from build123d import *

# Parameters (mm, degrees)
ESBO_O2_W                = 65.45
ESBO_O2_H                = 74.6
ESBO_O2_R                = 1.75
RESSALTO_EXTRUS_O1_DEPTH = 14.5
CORTE_EXTRUS_O1_REACH    = 84.743
ESBO_O3_W                = 6.5
ESBO_O3_H                = 12.9
ESBO_O4_W                = 48
ESBO_O4_H                = 74.6
RESSALTO_EXTRUS_O2_DEPTH = 4.5
ESBO_O5_W                = 20.2
ESBO_O5_H                = 12.15
ESBO_O5_W_2              = 30.35
RESSALTO_EXTRUS_O3_DEPTH = 8
ESBO_O6_R                = 4
RESSALTO_EXTRUS_O4_DEPTH = 12
FILETE1_R                = 0.8
CORTE_EXTRUS_O2_REACH    = 86.916
ESBO_O7_W                = 40.368182155
ESBO_O7_H                = 2.522042385
ESBO_O8_W                = 58.468294986
ESBO_O8_H                = 2.522042385
CORTE_EXTRUS_O3_DEPTH    = 71.953968353
ESBO_O9_W                = 3.722226521
ESBO_O9_H                = 2.522042385
ESBO_O9_W_2              = 3.909591324
CORTE_EXTRUS_O4_DEPTH    = 4
ESBO_O10_W               = 3.909591324
ESBO_O10_H               = 2.522042385
ESBO_O10_W_2             = 3.722226521
CORTE_EXTRUS_O5_DEPTH    = 3
FILETE2_R                = 1.5
FILETE3_R                = 0.3
ESBO_O11_W               = 9.960941138
ESBO_O11_H               = 18.14579458
RESSALTO_EXTRUS_O5_DEPTH = 6
ESBO_O12_W               = 18.14579458
ESBO_O12_H               = 6.154854005
CORTE_EXTRUS_O6_DEPTH    = 0.1
FILETE4_R                = 0.3


with BuildPart() as part:
    # Esboço2 → Ressalto-extrusão1 (new body)
    with BuildSketch(Plane(origin=(0, 0, 0), x_dir=(1, 0, 0), z_dir=(0, 1, 0))):
        Rectangle(ESBO_O2_W, ESBO_O2_H)
        with Locations(Location((27.725, 32.8, 0), (0, 0, 270))):
            Circle(ESBO_O2_R, mode=Mode.SUBTRACT)
        with Locations(Location((-27.725, 32.8, 0), (0, 0, 270))):
            Circle(ESBO_O2_R, mode=Mode.SUBTRACT)
        with Locations(Location((27.725, -32.8, 0), (0, 0, 270))):
            Circle(ESBO_O2_R, mode=Mode.SUBTRACT)
        with Locations(Location((-27.725, -32.8, 0), (0, 0, 270))):
            Circle(ESBO_O2_R, mode=Mode.SUBTRACT)
    extrude(amount=-RESSALTO_EXTRUS_O1_DEPTH)

    # Esboço3 → Corte-extrusão1 (cut, up to next)
    with BuildSketch(Plane(origin=(0, 0, -37.3), x_dir=(-1, 0, 0), z_dir=(0, 0, -1)), mode=Mode.PRIVATE) as corte_extrus_o1_sk1:
        with Locations((-27.975, -8.05)):
            Rectangle(ESBO_O3_W, ESBO_O3_H)
    corte_extrus_o1_tool1 = extrude(corte_extrus_o1_sk1.sketch, amount=-CORTE_EXTRUS_O1_REACH, mode=Mode.PRIVATE) & part.part
    # Esboço3 → Corte-extrusão1 (cut, up to next)
    with BuildSketch(Plane(origin=(0, 0, -37.3), x_dir=(-1, 0, 0), z_dir=(0, 0, -1)), mode=Mode.PRIVATE) as corte_extrus_o1_sk2:
        with Locations((-19.975, -8.05)):
            Rectangle(ESBO_O3_W, ESBO_O3_H)
    corte_extrus_o1_tool2 = extrude(corte_extrus_o1_sk2.sketch, amount=-CORTE_EXTRUS_O1_REACH, mode=Mode.PRIVATE) & part.part
    # Esboço3 → Corte-extrusão1 (cut, up to next)
    with BuildSketch(Plane(origin=(0, 0, -37.3), x_dir=(-1, 0, 0), z_dir=(0, 0, -1)), mode=Mode.PRIVATE) as corte_extrus_o1_sk3:
        with Locations((-11.975, -8.05)):
            Rectangle(ESBO_O3_W, ESBO_O3_H)
    corte_extrus_o1_tool3 = extrude(corte_extrus_o1_sk3.sketch, amount=-CORTE_EXTRUS_O1_REACH, mode=Mode.PRIVATE) & part.part
    # Esboço3 → Corte-extrusão1 (cut, up to next)
    with BuildSketch(Plane(origin=(0, 0, -37.3), x_dir=(-1, 0, 0), z_dir=(0, 0, -1)), mode=Mode.PRIVATE) as corte_extrus_o1_sk4:
        with Locations((-3.975, -8.05)):
            Rectangle(ESBO_O3_W, ESBO_O3_H)
    corte_extrus_o1_tool4 = extrude(corte_extrus_o1_sk4.sketch, amount=-CORTE_EXTRUS_O1_REACH, mode=Mode.PRIVATE) & part.part
    # Esboço3 → Corte-extrusão1 (cut, up to next)
    with BuildSketch(Plane(origin=(0, 0, -37.3), x_dir=(-1, 0, 0), z_dir=(0, 0, -1)), mode=Mode.PRIVATE) as corte_extrus_o1_sk5:
        with Locations((4.025, -8.05)):
            Rectangle(ESBO_O3_W, ESBO_O3_H)
    corte_extrus_o1_tool5 = extrude(corte_extrus_o1_sk5.sketch, amount=-CORTE_EXTRUS_O1_REACH, mode=Mode.PRIVATE) & part.part
    # Esboço3 → Corte-extrusão1 (cut, up to next)
    with BuildSketch(Plane(origin=(0, 0, -37.3), x_dir=(-1, 0, 0), z_dir=(0, 0, -1)), mode=Mode.PRIVATE) as corte_extrus_o1_sk6:
        with Locations((12.025, -8.05)):
            Rectangle(ESBO_O3_W, ESBO_O3_H)
    corte_extrus_o1_tool6 = extrude(corte_extrus_o1_sk6.sketch, amount=-CORTE_EXTRUS_O1_REACH, mode=Mode.PRIVATE) & part.part
    # Esboço3 → Corte-extrusão1 (cut, up to next)
    with BuildSketch(Plane(origin=(0, 0, -37.3), x_dir=(-1, 0, 0), z_dir=(0, 0, -1)), mode=Mode.PRIVATE) as corte_extrus_o1_sk7:
        with Locations((20.025, -8.05)):
            Rectangle(ESBO_O3_W, ESBO_O3_H)
    corte_extrus_o1_tool7 = extrude(corte_extrus_o1_sk7.sketch, amount=-CORTE_EXTRUS_O1_REACH, mode=Mode.PRIVATE) & part.part
    # Esboço3 → Corte-extrusão1 (cut, up to next)
    with BuildSketch(Plane(origin=(0, 0, -37.3), x_dir=(-1, 0, 0), z_dir=(0, 0, -1)), mode=Mode.PRIVATE) as corte_extrus_o1_sk8:
        with Locations((28.025, -8.05)):
            Rectangle(ESBO_O3_W, ESBO_O3_H)
    corte_extrus_o1_tool8 = extrude(corte_extrus_o1_sk8.sketch, amount=-CORTE_EXTRUS_O1_REACH, mode=Mode.PRIVATE) & part.part
    add(corte_extrus_o1_tool1.solids().sort_by_distance((27.975, -8.05, -37.3))[0], mode=Mode.SUBTRACT)
    add(corte_extrus_o1_tool2.solids().sort_by_distance((19.975, -8.05, -37.3))[0], mode=Mode.SUBTRACT)
    add(corte_extrus_o1_tool3.solids().sort_by_distance((11.975, -8.05, -37.3))[0], mode=Mode.SUBTRACT)
    add(corte_extrus_o1_tool4.solids().sort_by_distance((3.975, -8.05, -37.3))[0], mode=Mode.SUBTRACT)
    add(corte_extrus_o1_tool5.solids().sort_by_distance((-4.025, -8.05, -37.3))[0], mode=Mode.SUBTRACT)
    add(corte_extrus_o1_tool6.solids().sort_by_distance((-12.025, -8.05, -37.3))[0], mode=Mode.SUBTRACT)
    add(corte_extrus_o1_tool7.solids().sort_by_distance((-20.025, -8.05, -37.3))[0], mode=Mode.SUBTRACT)
    add(corte_extrus_o1_tool8.solids().sort_by_distance((-28.025, -8.05, -37.3))[0], mode=Mode.SUBTRACT)

    # Esboço4 → Ressalto-extrusão2 (add)
    with BuildSketch(Plane(origin=(0, 0, 0), x_dir=(1, 0, 0), z_dir=(0, 1, 0))):
        Rectangle(ESBO_O4_W, ESBO_O4_H)
    extrude(amount=RESSALTO_EXTRUS_O2_DEPTH)

    # Esboço5 → Ressalto-extrusão3 (add)
    with BuildSketch(Plane(origin=(0, 4.5, 0), x_dir=(1, 0, 0), z_dir=(0, 1, 0))):
        with Locations((0, 33.225)):
            Rectangle(ESBO_O5_W, ESBO_O5_H)
        with Locations((0, -33.225)):
            Rectangle(ESBO_O5_W_2, ESBO_O5_H)
    extrude(amount=RESSALTO_EXTRUS_O3_DEPTH)

    # Esboço6 → Ressalto-extrusão4 (add)
    with BuildSketch(Plane(origin=(0, 4.5, 0), x_dir=(1, 0, 0), z_dir=(0, 1, 0))):
        with Locations((20, -22.3)):
            Circle(ESBO_O6_R)
        with Locations(Location((4, -20.8, 0), (0, 0, 270))):
            Circle(ESBO_O6_R)
    extrude(amount=RESSALTO_EXTRUS_O4_DEPTH)

    # Filete1
    filete1_edges = [part.edges().sort_by_distance(p)[0] for p in [
        (16, 16.5, 22.3),
        (4, 16.5, 16.8),
    ]]
    fillet(filete1_edges, radius=FILETE1_R)

    # Esboço7 → Corte-extrusão2 (cut, up to next)
    with BuildSketch(Plane(origin=(0, 0, -37.3), x_dir=(-1, 0, 0), z_dir=(0, 0, -1)), mode=Mode.PRIVATE) as corte_extrus_o2_sk1:
        with Locations((0.093682401, 1.261021193)):
            Rectangle(ESBO_O7_W, ESBO_O7_H)
    corte_extrus_o2_tool1 = extrude(corte_extrus_o2_sk1.sketch, amount=-CORTE_EXTRUS_O2_REACH, mode=Mode.PRIVATE) & part.part
    add(corte_extrus_o2_tool1.solids().sort_by_distance((-0.093682, 1.261021, -37.3))[0], mode=Mode.SUBTRACT)

    # Esboço8 → Corte-extrusão3 (cut, through all)
    with BuildSketch(Plane.ZY.offset(24)):
        with Locations((-1.218876055, 1.261021193)):
            Rectangle(ESBO_O8_W, ESBO_O8_H)
    extrude(amount=-CORTE_EXTRUS_O3_DEPTH, mode=Mode.SUBTRACT)

    # Esboço9 → Corte-extrusão4 (cut)
    with BuildSketch(Plane.XY.offset(37.3)):
        with Locations((-22.13888674, 1.261021193)):
            Rectangle(ESBO_O9_W, ESBO_O9_H)
        with Locations((22.045204338, 1.261021193)):
            Rectangle(ESBO_O9_W_2, ESBO_O9_H)
    extrude(amount=-CORTE_EXTRUS_O4_DEPTH, mode=Mode.SUBTRACT)

    # Esboço10 → Corte-extrusão5 (cut)
    with BuildSketch(Plane(origin=(0, 0, -37.3), x_dir=(-1, 0, 0), z_dir=(0, 0, -1))):
        with Locations((-22.045204338, 1.261021193)):
            Rectangle(ESBO_O10_W, ESBO_O10_H)
        with Locations((22.13888674, 1.261021193)):
            Rectangle(ESBO_O10_W_2, ESBO_O10_H)
    extrude(amount=-CORTE_EXTRUS_O5_DEPTH, mode=Mode.SUBTRACT)

    # Filete2
    filete2_edges = [part.edges().sort_by_distance(p)[0] for p in [
        (24, 1.261021193, -30.453023548),
        (20.090408676, 1.261021193, -30.453023548),
        (-20.277773479, 1.261021193, -30.453023548),
        (24, 1.261021193, 28.015271438),
        (20.090408676, 1.261021193, 28.015271438),
        (-20.277773479, 1.261021193, 28.015271438),
        (-24, 1.261021193, -30.453023548),
        (-24, 1.261021193, 28.015271438),
        (-20.277773479, 1.261021193, 33.3),
        (-24, 1.261021193, 33.3),
        (20.090408676, 1.261021193, 33.3),
        (24, 1.261021193, 33.3),
        (20.090408676, 1.261021193, -34.3),
        (24, 1.261021193, -34.3),
        (-20.277773479, 1.261021193, -34.3),
        (-24, 1.261021193, -34.3),
    ]]
    fillet(filete2_edges, radius=FILETE2_R)

    # Filete3
    filete3_edges = [part.edges().sort_by_distance(p)[0] for p in [
        (-10.1, 8.5, -39.3),
        (-10.1, 8.5, -27.15),
        (10.1, 8.5, -27.15),
        (0, 4.5, -39.3),
        (10.1, 8.5, -39.3),
        (-10.1, 12.5, -33.225),
        (0, 12.5, -27.15),
        (10.1, 12.5, -33.225),
        (0, 12.5, -39.3),
        (15.175, 8.5, 39.3),
        (15.175, 8.5, 27.15),
        (-15.175, 8.5, 27.15),
        (0, 4.5, 39.3),
        (-15.175, 8.5, 39.3),
        (15.175, 12.5, 33.225),
        (0, 12.5, 27.15),
        (-15.175, 12.5, 33.225),
        (0, 12.5, 39.3),
    ]]
    fillet(filete3_edges, radius=FILETE3_R)

    # Esboço11 → Ressalto-extrusão5 (add)
    with BuildSketch(Plane(origin=(0, 4.5, 0), x_dir=(1, 0, 0), z_dir=(0, 1, 0))):
        with Locations((-19.019529431, -15.624104827)):
            Rectangle(ESBO_O11_W, ESBO_O11_H)
    extrude(amount=RESSALTO_EXTRUS_O5_DEPTH)

    # Esboço12 → Corte-extrusão6 (cut)
    with BuildSketch(Plane.ZY.offset(24)):
        with Locations((15.624104827, 7.422572997)):
            Rectangle(ESBO_O12_W, ESBO_O12_H)
    extrude(amount=-CORTE_EXTRUS_O6_DEPTH, mode=Mode.SUBTRACT)

    # Filete4
    filete4_edges = [part.edges().sort_by_distance(p)[0] for p in [
        (-14.039058862, 7.5, 24.697002117),
        (-14.039058862, 7.5, 6.551207537),
        (-14.039058862, 10.5, 15.624104827),
        (-18.969529431, 10.5, 6.551207537),
        (-18.969529431, 10.5, 24.697002117),
        (-23.9, 7.5, 6.551207537),
        (-23.9, 7.5, 24.697002117),
        (-23.9, 10.5, 15.624104827),
    ]]
    fillet(filete4_edges, radius=FILETE4_R)


solid = part.part
Can you work these out from the model? Positions are in its coordinate system, mm. A direction names the side the tool comes from. Round coordinates to 2 decimals unless told otherwise and drop trailing zeros. Loops run counter-clockwise (first coordinate to the right, second up) from the corner with the lowest first, then second, coordinate; pieces in that order, holes last. Notation, with made-up numbers: (17, -39) - (48, -39) arc R12 ccw to (48, -18) - close; hole circle Ø4 at (80, 50.25). An arc over 180 degrees is marked (long way). Use CSV: the item, a comma, the result in double quotes. Start each with the question number.
1) Please list where these lines run through material, in increasing order: probe 1 along X at (y, z) = (-0.7, -32.8) (3 decimals); probe 2 along Y at (x, z) = (-15.5, -3.5); probe 3 along Y at (x, z) = (20.5, 12.5). Write a range as [from, to].
2) If we section it at A-A on x = -4: Write out the boundary of the cut face in (y, z), plus the area to 3 significant figures.
3) If we section it at B-B on y = -7: Count the separate pieces of the cut face and the enclosed holes in it, plus the area to 3 significant figures.
4) For faces 1 (the flat face through (-19, 7, 6.551)), 2 (the flat face through (0, 0, -1)), 3 (the flat face through (0, 4, 37.3)), 4 (the flat face through (24.725, -8, -1)), 5 (the flat face through (-15.175, 8, 33)), which set-ups out of +Z, -Z, +X, -X, +Y, -Y let a thin tool reach every point of the face, with its end or its side?
5) We'd pull the mould along X, two halves only. Please class faces 6 (the flat face through (-14.039, 7, 16)), 7 (the flat face through (-10.1, 8, -33)), 8 (the flat face through (0, 8, 39.3)): released by +X, released by -X, zero draft, split by the parting line, or undercut.
6) For pin 1 Ø2 at (x, z) = (21, -11) entering from -Y; pin 2 Ø0.6 at (x, y) = (-22, 1) entering from +Z; pin 3 Ø2.5 at (y, z) = (9, 31.5) entering from +X (3 decimals), each with a flat end and sliding along its axis, tell me the tip position at first contact or that it passes through.
Geometry results:
1,probe 1,"x = [-32.725, -29.475], [-25.975, 25.975], [29.475, 32.725]"
1,probe 2,"y = [-14.5, 0], [2.52, 4.5]"
1,probe 3,"y = [-1.6, 0], [2.52, 4.5]"
2,outline,"(-1.6, -37.3) - (0, -37.3) - (0, 37.3) - (-1.6, 37.3) - close; (2.52, -37.3) - (4.5, -37.3) - (4.5, -39) arc R0.3 ccw to (4.8, -39.3) - (12.2, -39.3) arc R0.3 ccw to (12.5, -39) - (12.5, -27.45) arc R0.3 ccw to (12.2, -27.15) - (4.5, -27.15) - (4.5, 27.15) - (12.2, 27.15) arc R0.3 ccw to (12.5, 27.45) - (12.5, 39) arc R0.3 ccw to (12.2, 39.3) - (4.8, 39.3) arc R0.3 ccw to (4.5, 39) - (4.5, 37.3) - (2.52, 37.3) - close"
2,area,"461 mm2"
3,separate pieces,"9"
3,enclosed holes,"0"
3,area,"1,000 mm2"
4,face 1,"-Z, +X, -X, +Y"
4,face 2,"none"
4,face 3,"+Z, +X, -X, -Y"
4,face 4,"+Z, -Z, -Y"
4,face 5,"+Z, -X, +Y"
5,face 6,"undercut"
5,face 7,"released by -X"
5,face 8,"zero draft"
6,pin 1,"stops at y = -1.6"
6,pin 2,"stops at z = 33.3"
6,pin 3,"stops at x = 15.175"
